from build123d import *

# Parameters (mm, degrees)
BOSS_EXTRUDE1_DEPTH           = 510
CHAMFER6_SIZE                 = 31.75
CHAMFER7_SIZE                 = 31.75
TOPHOLES_SKETCH3_R            = 1.5875
TOPHOLES_CUT_EXTRUDE2_DEPTH   = 512.785690622
FRONTHOLES_SKETCH4_R          = 1.5875
FRONTHOLES_CUT_EXTRUDE3_DEPTH = 512.785690622


with BuildPart() as part:
    # Sketch1 → Boss-Extrude1 (new body)
    with BuildSketch(Plane(origin=(0, 0, 0), x_dir=(0, 0, -1), z_dir=(1, 0, 0))):
        Polygon((0, 0), (-31.75, 0), (-31.75, 3.175), (-3.175, 3.175), (-3.175, 31.75), (0, 31.75), align=None)
    extrude(amount=BOSS_EXTRUDE1_DEPTH)

    # Chamfer6
    chamfer6_edges = [part.edges().sort_by_distance(p)[0] for p in [
        (510, 1.5875, 31.75),
    ]]
    chamfer(chamfer6_edges, length=CHAMFER6_SIZE - 0.0001)  # a hair under: the kernel refuses the full size

    # Chamfer7
    chamfer7_edges = [part.edges().sort_by_distance(p)[0] for p in [
        (0, 1.5875, 31.75),
    ]]
    chamfer(chamfer7_edges, length=CHAMFER7_SIZE - 0.0001)  # a hair under: the kernel refuses the full size

    # TopHoles-Sketch3 → TopHoles-Cut-Extrude2 (cut, through all)
    with BuildSketch(Plane(origin=(0, 3.175, 0), x_dir=(1, 0, 0), z_dir=(0, 1, 0))):
        with Locations(Location((58.7375, -23.8125, 0), (0, 0, 270))):
            Circle(TOPHOLES_SKETCH3_R)
        with Locations(Location((451.2625, -23.8125, 0), (0, 0, 270))):
            Circle(TOPHOLES_SKETCH3_R)
        with Locations(Location((451.2625, -11.1125, 0), (0, 0, 270))):
            Circle(TOPHOLES_SKETCH3_R)
        with Locations(Location((58.7375, -11.1125, 0), (0, 0, 270))):
            Circle(TOPHOLES_SKETCH3_R)
        with Locations(Location((486.1875, -11.1125, 0), (0, 0, 270))):
            Circle(TOPHOLES_SKETCH3_R)
        with Locations(Location((23.8125, -11.1125, 0), (0, 0, 270))):
            Circle(TOPHOLES_SKETCH3_R)
        with Locations(Location((127.5, -11.1125, 0), (0, 0, 270))):
            Circle(TOPHOLES_SKETCH3_R)
        with Locations(Location((255, -11.1125, 0), (0, 0, 270))):
            Circle(TOPHOLES_SKETCH3_R)
        with Locations(Location((382.5, -11.1125, 0), (0, 0, 270))):
            Circle(TOPHOLES_SKETCH3_R)
    extrude(amount=-TOPHOLES_CUT_EXTRUDE2_DEPTH, mode=Mode.SUBTRACT)

    # FrontHoles-Sketch4 → FrontHoles-Cut-Extrude3 (cut, through all)
    with BuildSketch(Plane.XY.offset(3.175)):
        with Locations((11.1125, 23.8125)):
            Circle(FRONTHOLES_SKETCH4_R)
        with Locations((489.3625, 23.8125)):
            Circle(FRONTHOLES_SKETCH4_R)
        with Locations((20.6375, 23.8125)):
            Circle(FRONTHOLES_SKETCH4_R)
        with Locations((498.8875, 23.8125)):
            Circle(FRONTHOLES_SKETCH4_R)
        with Locations((11.1125, 11.1125)):
            Circle(FRONTHOLES_SKETCH4_R)
        with Locations((20.6375, 11.1125)):
            Circle(FRONTHOLES_SKETCH4_R)
        with Locations((489.3625, 11.1125)):
            Circle(FRONTHOLES_SKETCH4_R)
        with Locations((498.8875, 11.1125)):
            Circle(FRONTHOLES_SKETCH4_R)
        with Locations((127.5, 11.1125)):
            Circle(FRONTHOLES_SKETCH4_R)
        with Locations((255, 11.1125)):
            Circle(FRONTHOLES_SKETCH4_R)
        with Locations((382.5, 11.1125)):
            Circle(FRONTHOLES_SKETCH4_R)
    extrude(amount=-FRONTHOLES_CUT_EXTRUDE3_DEPTH, mode=Mode.SUBTRACT)


solid = part.part
Check sheet for the modelled part. Datum: model origin and axes. Units: mm. A direction names the side the tool comes from. Round coordinates to 2 decimals unless told otherwise and drop trailing zeros. Loops run counter-clockwise (first coordinate to the right, second up) from the corner with the lowest first, then second, coordinate; pieces in that order, holes last. Notation, with made-up numbers: (-20.5, 43.25) - (-6.5, 43.25) arc R26 cw to (-6.5, 58.25) - close; hole circle Ø11 at (-36, 20). An arc over 180 degrees is marked (long way). Answer as CSV lines item,"result". Start each with the question number.
Item 1: Set-up check for faces 1 (the flat face through (251, 0, 16)), 2 (the flat face through (251, 17, 3.175)): record each of +Z, -Z, +X, -X, +Y, -Y from which the full face is reachable in a straight line by a thin tool's end or side.
Item 2: Depth check by flat-ended pin: P1, Ø2.5, axis at x = 58.74, z = 23.81, coming from the +Y side; P2, Ø10, axis at x = 147, y = 19, coming from the +Z side (3 decimals); P3, Ø4, axis at x = 127.5, z = 11.11, coming from the +Y side (3 decimals); P4, Ø2, axis at y = 4, z = 7.5, coming from the +X side. Enter the tip coordinate at first touch or a pass-through.
Item 3: Section check B-B (z = 17.5). Record the boundary of the cut face in (x, y) (3 decimals), and give its area (3 significant figures).
Item 4: Scan lines: line 1 (Y direction, x = 255, z = 1) (3 decimals); line 2 (Z direction, x = 127, y = 1); line 3 (Z direction, x = 41, y = 6.5) (3 decimals). Record each from-to range of solid material in increasing order. Write a range as [from, to].
Item 5: Section check A-A (x = 295). Record the boundary of the cut face in (y, z) (3 decimals).
Report:
1,face 1,"+Z, -Z, +X, -X, -Y"
1,face 2,"+Z, +X, -X, +Y"
2,P1,"passes through"
2,P2,"stops at z = 3.175"
2,P3,"stops at y = 3.175"
2,P4,"stops at x = 503.07"
3,outline,"(17.5, 0) - (492.5, 0) - (492.5, 3.175) - (17.5, 3.175) - close"
3,area,"1,510 mm2"
4,line 1,"y = [0, 9.525], [12.7, 31.75]"
4,line 2,"z = [0, 9.61], [12.62, 31.75]"
4,line 3,"z = [0, 3.175]"
5,outline,"(0, 0) - (31.75, 0) - (31.75, 3.175) - (3.175, 3.175) - (3.175, 31.75) - (0, 31.75) - close"
